CAD build for the part. Positions are in the model's coordinates, mm. Give positions to 0.01 mm unless a question says otherwise; leave off trailing zeros. Write each loop counter-clockwise with the first axis right and the second up, starting at its lowest first coordinate (ties: lowest second). Pieces come first, ordered by that corner, then holes. Notation, with made-up numbers: (24.5, 18) - (83.5, 18) arc R16 cw to (83.5, 32) - close; hole circle Ø11 at (-38.75, 4). An arc over 180 degrees is marked (long way). Put each result on its own line as item: value. Start each with the question number.
1. Cut at A-A on y = 0.7. List the corners of the cut face in (x, z), and give its area (3 significant figures).
2. Wall check: line 1 (Z direction, x = -10, y = 0.25); line 2 (X direction, y = 0.2, z = 22); line 3 (Z direction, x = -11, y = 0.6). Give the ranges that are in metal, low to high.
3. Mould opens along X. For faces 1 (the cylindrical face through (24.5, 0.51, -12.56)), 2 (the cylindrical face through (-10.987, 0.493, -9.678)), 3 (the flat face through (5, 0, 7)) say: +X half, -X half, draft (parallel to the pull), parting line (faces both ways), or undercut.
4. Cut at B-B on x = 20.5. List the corners of the cut face in (y, z).
Autodesk Inventor part; units mm, degrees
ref_plane "YZ Plane" through (0, 0, 0) normal (1, 0, 0) x (0, 1, 0)
ref_plane "XZ Plane" through (0, 0, 0) normal (0, 1, 0) x (-1, 0, 0)
ref_plane "XY Plane" through (0, 0, 0) normal (0, 0, 1) x (1, 0, 0)
sketch "Sketch1" plane through (0, 0, 0) normal (0, 1, 0) x (-1, 0, 0)
  line L0 (14.9302, 26.8372) -> (-25.0698, 26.8372)
  line L1 (-25.0698, 26.8372) -> (-25.0698, -13.1628)
  line L2 (-25.0698, -13.1628) -> (14.9302, -13.1628)
  line L3 (14.9302, -13.1628) -> (14.9302, 26.8372)
  line L4 (-5.0698, 26.8372) -> (-5.0698, -13.1628)
  line L5 (14.9302, 6.8372) -> (-25.0698, 6.8372)
  circle A0 centre (10.1802, -8.4128) radius 1.5
  circle A1 centre (10.1802, 22.0872) radius 1.5
  circle A2 centre (-20.3198, 22.0872) radius 1.5
  circle A3 centre (-20.3198, -8.4128) radius 1.5
  point P0 (0, 0)
  dimension "d0" = 40
  dimension "d1" = 40
  dimension "d2" = 3
  dimension "d3" = 3
  dimension "d4" = 3
  dimension "d5" = 3
  dimension "d6" = 30.5
  dimension "d7" = 30.5
  dimension "d8" = 30.5
  dimension "d9" = 30.5
  dimension "d10" = 15.25
  dimension "d11" = 15.25
  dimension "d12" = 15.25
  dimension "d13" = 15.25
extrude "Extrusion1" add sketch "Sketch1" along normal blind 1
fillet "Fillet1" radius 2 4 edges at (-14.9302, 0.5, 26.8372) (25.0698, 0.5, 26.8372) (25.0698, 0.5, -13.1628) (-14.9302, 0.5, -13.1628)
properties part number "CHIP"
Report:
1. outline: (-14.93, -11.16) arc R2 ccw to (-12.93, -13.16) - (23.07, -13.16) arc R2 ccw to (25.07, -11.16) - (25.07, 24.84) arc R2 ccw to (23.07, 26.84) - (-12.93, 26.84) arc R2 ccw to (-14.93, 24.84) - close; hole circle Ø3 at (-10.18, -8.41); hole circle Ø3 at (-10.18, 22.09); hole circle Ø3 at (20.32, -8.41); hole circle Ø3 at (20.32, 22.09)
1. area: 1,570 mm²
2. line 1: z = -13.16 to -9.9, -6.92 to 20.6, 23.58 to 26.84
2. line 2: x = -14.93 to -11.68, -8.68 to 18.82, 21.82 to 25.07
2. line 3: z = -13.16 to -9.67, -7.16 to 20.83, 23.34 to 26.84
3. face 1: +X half
3. face 2: undercut
3. face 3: draft
4. outline: (0, -13.16) - (1, -13.16) - (1, -9.9) - (0, -9.9) - close; (0, -6.92) - (1, -6.92) - (1, 20.6) - (0, 20.6) - close; (0, 23.58) - (1, 23.58) - (1, 26.84) - (0, 26.84) - close
